Input: part model. Units: mm. Frame: model coordinates. A direction names the side the tool comes from. Give positions to 0.01 mm unless a question says otherwise; leave off trailing zeros. Loops run counter-clockwise (first coordinate to the right, second up) from the corner with the lowest first, then second, coordinate; pieces in that order, holes last. Notation, with made-up numbers: (-4.5, 61.25) - (36.5, 61.25) arc R23 cw to (36.5, 76.25) - close; hole circle Ø2 at (-37.75, -14). An arc over 180 degrees is marked (long way). One line per question, with ' | ' between items. Start each with the question number.
from build123d import *

# Parameters (mm, degrees)
F1_DEPTH = 5
F2_R     = 2
F3_R     = 2
F4_R     = 2


with BuildPart() as f1:
    # F0 (on Top) → F1 (new body)
    with BuildSketch(Plane.XY):
        Polygon((69, 30), (69, 50), (-120, 50), (-120, 30), (-105, 45), (-105, 25), (-105, 5), (-120, 20), (-120, 0), (-120, -20), (-105, -5), (-105, -25), (-105, -45), (-120, -30), (-120, -50), (-90, -50), (-90, 0), (-87, 0), (-87, -50), (-27, -50), (-27, 0), (-24, 0), (-24, -50), (36, -50), (36, 0), (39, 0), (39, -50), (69, -50), (69, -30), (69, -29), (83.000012, -43.000012), (83.000012, -6.999988), (69, -21), (69, -20), (69, 0), (69, 20), (69, 21), (83.000012, 6.999988), (83.000012, 25), (83.000012, 43.000012), (69, 29), align=None)
    extrude(amount=F1_DEPTH)

    # F2
    f2_edges = [f1.edges().sort_by_distance(p)[0] for p in [
        (-105, 45, 2.5),
        (-105, 5, 2.5),
        (-105, -5, 2.5),
        (-105, -45, 2.5),
        (-120, -20, 2.5),
        (-120, -30, 2.5),
        (-120, 20, 2.5),
        (-120, 30, 2.5),
    ]]
    fillet(f2_edges, radius=F2_R)

    # F3
    f3_edges = [f1.edges().sort_by_distance(p)[0] for p in [
        (83.000012, 43.000012, 2.5),
        (83.000012, 6.999988, 2.5),
        (83.000012, -6.999988, 2.5),
        (83.000012, -43.000012, 2.5),
    ]]
    fillet(f3_edges, radius=F3_R)

    # F4
    f4_edges = [f1.edges().sort_by_distance(p)[0] for p in [
        (69, 21, 2.5),
        (69, 29, 2.5),
        (69, -21, 2.5),
        (69, -29, 2.5),
    ]]
    fillet(f4_edges, radius=F4_R)


solid = f1.part
Q1. Section A-A, the plane y = -27. Output: boundary loops of the cut face in (x, z), plus the area to 3 significant figures.
Q2. Line query: L1, parallel to X at y = -5, z = 0.85; L2, parallel to X at y = -19.5, z = 4.7; L3, parallel to X at y = -39, z = 1.25. Output: solid intervals per line, ascending. Write a range as from..to.
Q3. Access query for faces 1 (the face through (-90, -25, 2)), 2 (the face through (69, 42, 2)), 3 (the face through (-106.204, 7.994, 2.535)), 4 (the face through (-20, 1, 0)). Directions: +Z, -Z, +X, -X, +Y, -Y. A direction counts if a zero-diameter tool reaches every point of the face in a straight line with its end or side. Return the directions, or none.
Q4. Section C-C, the plane y = 22. Output: boundary loops of the cut face in (x, z).
Q5. First-contact query: pin 1 (2.5 mm diameter, centred on y = 40.5, z = 3.5, fed in from +X); pin 2 (0.9 mm diameter, centred on x = -26, z = 3.5, fed in from -Y); pin 3 (1.5 mm diameter, centred on y = 39, z = 2.5, fed in from +X); pin 4 (2.5 mm diameter, centred on y = -40, z = 2, fed in from +X). Flat tips, straight axial feed; report the tip coordinate or a pass-through.
Q6. Section B-B, the plane y = -5. Output: boundary loops of the cut face in (x, z).
Q7. Draft query along X for faces 5 (the face through (39, -25, 2)), 6 (the face through (-105, -50, 2)), 7 (the face through (83, 25, 2)). Return one class per face: +X half, -X half, draft (parallel to the pull), parting line (faces both ways), or undercut.
Solved:
1) outline: (-105, 0) - (-90, 0) - (-90, 5) - (-105, 5) - close; (-87, 0) - (-27, 0) - (-27, 5) - (-87, 5) - close; (-24, 0) - (36, 0) - (36, 5) - (-24, 5) - close; (39, 0) - (83, 0) - (83, 5) - (39, 5) - close | area: 895 mm²
2) L1: x = -120..-90, -87..-27, -24..36, 39..69 | L2: x = -105..-90, -87..-27, -24..36, 39..83 | L3: x = -120..-111, -105..-90, -87..-27, -24..36, 39..69, 79..82.82
3) face 1: +Z, -Z, -Y | face 2: +Z, -Z, +Y | face 3: +Z, -Z | face 4: -Z, +X, -X, +Y, -Y
4) outline: (-105, 0) - (83, 0) - (83, 5) - (-105, 5) - close
5) pin 1: stops at x = 82.68 | pin 2: stops at y = 0 | pin 3: stops at x = 83 | pin 4: stops at x = 82.91
6) outline: (-120, 0) - (-90, 0) - (-90, 5) - (-120, 5) - close; (-87, 0) - (-27, 0) - (-27, 5) - (-87, 5) - close; (-24, 0) - (36, 0) - (36, 5) - (-24, 5) - close; (39, 0) - (69, 0) - (69, 5) - (39, 5) - close
7) face 5: undercut | face 6: draft | face 7: +X half
